Geometry: final body of the model. Coordinates: model frame, mm. A direction names the side the tool comes from. Round coordinates to 2 decimals unless told otherwise and drop trailing zeros. Loops run counter-clockwise (first coordinate to the right, second up) from the corner with the lowest first, then second, coordinate; pieces in that order, holes last. Notation, with made-up numbers: (-25, -37) - (-12, -37) arc R18 cw to (-12, -12) - close; hole circle Ø1 at (-1, 0.25). An arc over 180 degrees is marked (long way). Answer as a JSON object with one key per item and string values. Group by question number.
Item 1: Line query: line 1 (X direction, y = 58.5, z = 65); line 2 (X direction, y = 56.1, z = 45); line 3 (Z direction, x = 175.25, y = 58.55). Output: solid intervals per line, ascending.
Item 2: Section B-B (z = 10). Return the cut outline in (x, y), plus the area to 3 significant figures.
Item 3: Section A-A (z = 45). Return the cut outline in (x, y), plus the area to 3 significant figures.
Item 4: Reachability of faces 4 (the face through (177, 58, 0)), 5 (the face through (175, 56.856, 6)) from +Z, -Z, +X, -X, +Y, -Y: full face, straight path, thin tool, end or side. Return the list, or none.
Item 5: Draft query along Z for faces 1 (the face through (177, 54.86, 37)), 2 (the face through (177, 58, 75)), 3 (the face through (175, 56.856, 26)). Return one class per face: released by +Z, released by -Z, zero draft, split by the parting line, or undercut.
Item 6: First-contact query: pin 1 (1.8 mm diameter, centred on x = 176, z = 46, fed in from +Y). Flat tip, straight axial feed; report the tip coordinate or a pass-through.
Item 7: Section C-C (x = 177.5). Count the separate pieces of the cut face and the enclosed holes in it, plus the area to 3 significant figures.
```python
from build123d import *

# Parameters (mm, degrees)
EXTRUDE_1_DEPTH              = 75
HOLE_WIZARD_M6_1_D           = 3.5
HOLE_WIZARD_M6_1_DEPTH       = 5.495410489
HOLE_WIZARD_M6_1_CBORE_D     = 6
HOLE_WIZARD_M6_1_CBORE_DEPTH = 3.5


with BuildPart() as part:
    # Model → 凸台-拉伸1 (new body)
    with BuildSketch(Plane.XY):
        Polygon((172.467003798, 54.860433324), (176.62288374, 54.860433324), (180.778763681, 54.860433324), (181.122753743, 55.174540135), (181.122753743, 57.578663559), (180.378777275, 58.313663309), (179.814791529, 58.313663309), (179.814791529, 58.850465041), (180.366775583, 58.850465041), (181.122753743, 59.563028946), (181.122753743, 60.355843813), (176.62288374, 60.355843813), (172.123013736, 60.355843813), (172.123013736, 59.563028946), (172.878991897, 58.850465041), (173.43097595, 58.850465041), (173.43097595, 58.313663309), (172.866992243, 58.313663309), (172.123013736, 57.578663559), (172.123013736, 55.174540135), align=None)
    extrude(amount=EXTRUDE_1_DEPTH)

    # M6 六角头螺栓的柱形沉头孔1
    with Locations(Plane(origin=(176.62288374, 60.355843813, 5), x_dir=(0, 0, 1), z_dir=(0, 1, 0))):
        with Locations((0, 0), (20, 0), (40, 0), (60, 0)):
            CounterBoreHole(HOLE_WIZARD_M6_1_D / 2, HOLE_WIZARD_M6_1_CBORE_D / 2, HOLE_WIZARD_M6_1_CBORE_DEPTH, depth=HOLE_WIZARD_M6_1_DEPTH)


solid = part.part
```
Values:
{
 "1": {"line 1": "x = 173.43 to 173.62, 179.62 to 179.81", "line 2": "x = 172.12 to 174.87, 178.37 to 181.12", "line 3": "z = 0 to 2.33, 7.67 to 22.33, 27.67 to 42.33, 47.67 to 62.33, 67.67 to 75"},
 "2": {"outline": "(172.12, 55.17) - (172.47, 54.86) - (180.78, 54.86) - (181.12, 55.17) - (181.12, 57.58) - (180.38, 58.31) - (179.81, 58.31) - (179.81, 58.85) - (180.37, 58.85) - (181.12, 59.56) - (181.12, 60.36) - (172.12, 60.36) - (172.12, 59.56) - (172.88, 58.85) - (173.43, 58.85) - (173.43, 58.31) - (172.87, 58.31) - (172.12, 57.58) - close", "area": "46.9 mm^2"},
 "3": {"outline": "(172.12, 55.17) - (172.47, 54.86) - (174.87, 54.86) - (174.87, 56.86) - (173.62, 56.86) - (173.62, 60.36) - (172.12, 60.36) - (172.12, 59.56) - (172.88, 58.85) - (173.43, 58.85) - (173.43, 58.31) - (172.87, 58.31) - (172.12, 57.58) - close; (178.37, 54.86) - (180.78, 54.86) - (181.12, 55.17) - (181.12, 57.58) - (180.38, 58.31) - (179.81, 58.31) - (179.81, 58.85) - (180.37, 58.85) - (181.12, 59.56) - (181.12, 60.36) - (179.62, 60.36) - (179.62, 56.86) - (178.37, 56.86) - close", "area": "18.9 mm^2"},
 "4": {"face 4": "-Z, +X, -X, +Y, -Y", "face 5": "+Y"},
 "5": {"face 1": "zero draft", "face 2": "released by +Z", "face 3": "undercut"},
 "6": {"pin 1": "stops at y = 56.86"},
 "7": {"separate pieces": "5", "enclosed holes": "0", "area": "308 mm^2"}
}
